Design review of the part built by this model. Coordinates are the model's own, in mm. Face numbers are marked on the shaded views. A direction names the side the tool comes from. Round coordinates to 2 decimals unless told otherwise and drop trailing zeros. Write each loop counter-clockwise with the first axis right and the second up, starting at its lowest first coordinate (ties: lowest second). Pieces come first, ordered by that corner, then holes. Notation, with made-up numbers: (35, 31) -> (67, 31) arc R21 cw to (67, 35) -> close; hole circle Ø8 at (83.5, 34). An arc over 180 degrees is marked (long way). Write item = value, one per line. Start each with the question number.
Item 1: Add section B-B, the plane y = -17.5. State the section outline as (x, z) points.
Item 2: Machinability: for the marked faces 1, 2, 3 and 4, which of the approach directions +Z, -Z, +X, -X, +Y, -Y give a long, thin tool a straight path to every point of the face, cutting with its end or side? Answer none if there is none.
Item 3: For pin 1 Ø7 at (x, z) = (32, 16) entering from -Y; pin 2 Ø1.5 at (y, z) = (15, -4.5) entering from -X; pin 3 Ø1 at (x, y) = (0, -14.5) entering from -Z; pin 4 Ø6 at (y, z) = (1, 7.5) entering from +X, all flat-tipped, find the tip position at first contact; note any pin that passes through.
Item 4: To check wall thickness, follow L1, parallel to X at y = 6.2, z = 18.1; L2, parallel to Z at x = -13, y = -14; L3, parallel to X at y = 4.5, z = 19.5. State the ranges of each line that lie inside material, in increasing order.
Item 5: Add section C-C, the plane z = -4. State the section outline as (x, y) points, then the cut area to 3 significant figures.
Item 6: Add section A-A, the plane z = 18.1. State the section outline as (x, y) points.
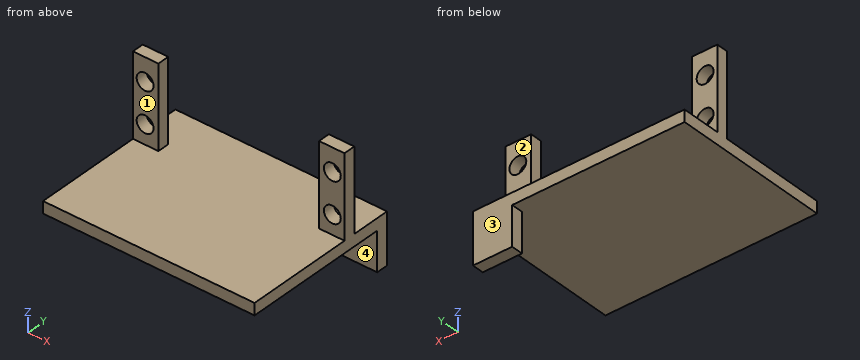
from build123d import *

# Parameters (mm, degrees)
SKETCH1_W           = 54
SKETCH1_H           = 40.5
BOSS_EXTRUDE1_DEPTH = 3
SKETCH3_W           = 6.5
SKETCH3_H           = 3
BOSS_EXTRUDE2_DEPTH = 21
SKETCH4_W           = 10
SKETCH4_H           = 3
BOSS_EXTRUDE3_DEPTH = 10
SKETCH5_R           = 2.15
CUT_EXTRUDE1_DEPTH  = 3


with BuildPart() as part:
    # Sketch1 → Boss-Extrude1 (new body)
    with BuildSketch(Plane.XY):
        with Locations((7.441119081, -3.357474474)):
            Rectangle(SKETCH1_W, SKETCH1_H)
    extrude(amount=BOSS_EXTRUDE1_DEPTH)

    # Sketch3 → Boss-Extrude2 (add)
    with BuildSketch(Plane.XY.offset(3)):
        with Locations((31.191119081, 5.392525526)):
            Rectangle(SKETCH3_W, SKETCH3_H)
        with Locations((-16.308880919, 5.392525526)):
            Rectangle(SKETCH3_W, SKETCH3_H)
    extrude(amount=BOSS_EXTRUDE2_DEPTH)

    # Sketch4 → Boss-Extrude3 (add)
    with BuildSketch(Plane(origin=(0, 0, 0), x_dir=(-1, 0, 0), z_dir=(0, 0, -1))):
        with Locations((-29.441119081, 15.392525526)):
            Rectangle(SKETCH4_W, SKETCH4_H)
    extrude(amount=BOSS_EXTRUDE3_DEPTH)

    # Sketch5 → Cut-Extrude1 (cut)
    with BuildSketch(Plane(origin=(0, 6.892525526, 0), x_dir=(1, 0, 0), z_dir=(0, 1, 0))):
        with Locations(Location((31.341119081, -18.1, 0), (0, 0, 270))):
            Circle(SKETCH5_R)
        with Locations(Location((31.341119081, -7.9, 0), (0, 0, 270))):
            Circle(SKETCH5_R)
        with Locations(Location((-16.458880919, -18.1, 0), (0, 0, 270))):
            Circle(SKETCH5_R)
        with Locations(Location((-16.458880919, -7.9, 0), (0, 0, 270))):
            Circle(SKETCH5_R)
    extrude(amount=-CUT_EXTRUDE1_DEPTH, mode=Mode.SUBTRACT)


solid = part.part
Result set:
q1.outline = (-19.56, 0) -> (34.44, 0) -> (34.44, 3) -> (-19.56, 3) -> close
q2.face_1 = +Z, +X, -X, -Y
q2.face_2 = +Z, +X, -X, +Y
q2.face_3 = +Z, -Z, +X, -X, +Y
q2.face_4 = -Z, +X, -X, -Y
q3.pin_1 = 3.89
q3.pin_2 = 24.44
q3.pin_3 = 0
q3.pin_4 = 34.44
q4.L1 = -19.56 to -18.61, -14.31 to -13.06, 27.94 to 29.19, 33.49 to 34.44
q4.L2 = 0 to 3
q4.L3 = -19.56 to -18.09, -14.83 to -13.06, 27.94 to 29.71, 32.97 to 34.44
q5.outline = (24.44, 13.89) -> (34.44, 13.89) -> (34.44, 16.89) -> (24.44, 16.89) -> close
q5.area = 30.0 mm²
q6.outline = (-19.56, 3.89) -> (-18.61, 3.89) -> (-18.61, 6.89) -> (-19.56, 6.89) -> close; (-14.31, 3.89) -> (-13.06, 3.89) -> (-13.06, 6.89) -> (-14.31, 6.89) -> close; (27.94, 3.89) -> (29.19, 3.89) -> (29.19, 6.89) -> (27.94, 6.89) -> close; (33.49, 3.89) -> (34.44, 3.89) -> (34.44, 6.89) -> (33.49, 6.89) -> close
